```python
from build123d import *

# Parameters (mm, degrees)
BOSS_EXTRU_1_DEPTH  = 40
SKETCH1_R           = 2
CUT_EXTRUDE1_DEPTH  = 29
SKETCH2_W           = 15
SKETCH2_H           = 9
BOSS_EXTRUDE1_DEPTH = 6


with BuildPart() as part:
    # Esquisse1 → Boss.-Extru.1 (new body)
    with BuildSketch(Plane.XY):
        Polygon((0, 0), (-15, 0), (-15, -6), (0, -6), (0, -41), (-15, -41), (-15, -56), (20.126965986, -56), (20.126965986, -41), (10.126965986, -41), (10.126965986, 0), align=None)
    extrude(amount=BOSS_EXTRU_1_DEPTH)

    # Sketch1 → Cut-Extrude1 (cut)
    with BuildSketch(Plane(origin=(0, -41, 0), x_dir=(1, 0, 0), z_dir=(0, 1, 0))):
        with Locations(Location((15.126965986, -8, 0), (0, 0, 270))):
            Circle(SKETCH1_R)
        with Locations(Location((15.126965986, -32, 0), (0, 0, 270))):
            Circle(SKETCH1_R)
    extrude(amount=-CUT_EXTRUDE1_DEPTH, mode=Mode.SUBTRACT)

    # Sketch2 → Boss-Extrude1 (add)
    with BuildSketch(Plane.XY.offset(40)):
        with Locations((-7.5, -36.5)):
            Rectangle(SKETCH2_W, SKETCH2_H)
    extrude(amount=-BOSS_EXTRUDE1_DEPTH)


solid = part.part
```
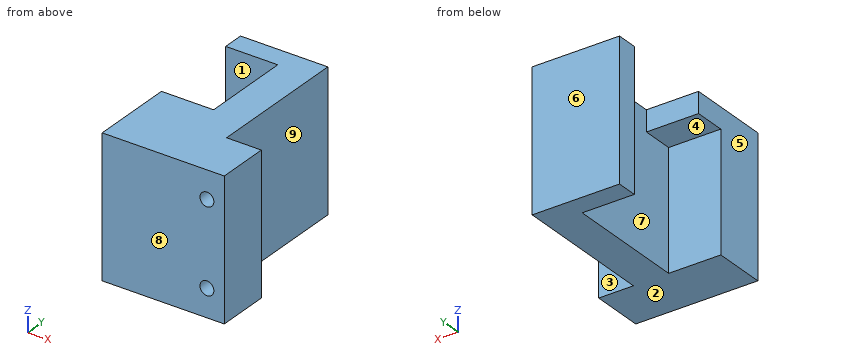
Check sheet for the modelled part. Datum: model origin and axes. Units: mm. Face numbers are marked on the shaded views. A direction names the side the tool comes from. Give positions to 0.01 mm unless a question says otherwise; leave off trailing zeros. Order: outer loops, then holes, each group sorted by start corner. A loop starts at its lowest first (then second) coordinate and runs counter-clockwise, first axis right, second up. Notation, with made-up numbers: M 8,43.5 L 34,43.5 A11 cw 34,63.5 Z; hole C 86,-8.5 d11. An arc over 180 degrees is marked long. Answer in a Markdown table with one row per item.
1) Cross-section at D-D, the plane y = -35.5. Enter the section's corners in (x, z), plus the area to 3 significant figures.
Filled sheet:
| item | result |
|---|---|
| outline | M -15,34 L 0,34 L 0,0 L 10.13,0 L 10.13,40 L -15,40 Z |
| area | 495 mm2 |
2) Cross-section at A-A, the plane x = -4.5. Enter the section's corners in (y, z), plus the area to 3 significant figures.
Filled sheet:
| item | result |
|---|---|
| outline | M -56,0 L -41,0 L -41,34 L -32,34 L -32,40 L -56,40 Z; M -6,0 L 0,0 L 0,40 L -6,40 Z |
| area | 894 mm2 |
3) Release check for a two-part mould opening along Y. For the marked faces 6, 7, 8 and 9 record: +Y half, -Y half, draft (parallel to the pull), parting line (faces both ways), or undercut.
Filled sheet:
| item | result |
|---|---|
| face 6 | +Y half |
| face 7 | undercut |
| face 8 | -Y half |
| face 9 | draft |
4) Access from +Z, -Z, +X, -X, +Y, -Y to the whole of each face (thin tool, end or side, straight path). Record for the marked faces 1, 2, 3, 4 and 5.
Filled sheet:
| item | result |
|---|---|
| face 1 | +Z, -Z, -X |
| face 2 | -Z, +X, -X, +Y, -Y |
| face 3 | +Z, -Z, +X, +Y |
| face 4 | -Z, -X |
| face 5 | +Z, -Z, -X, +Y, -Y |
5) Gauge pin test, flat ends, axial feed: P1, Ø1.5, axis at x = 12.5, z = 17.5, coming from the +Y side; P2, Ø1, axis at x = 11, y = -6.5, coming from the +Z side; P3, Ø7, axis at x = -10.5, y = -36, coming from the -Z side; P4, Ø8, axis at y = -16.5, z = 15.5, coming from the -X side. Record the tip position at first contact, or that the pin passes through.
Filled sheet:
| item | result |
|---|---|
| P1 | stops at y = -41 |
| P2 | passes through |
| P3 | stops at z = 34 |
| P4 | stops at x = 0 |
6) Thickness scan on L1, parallel to Y at x = -3, z = 5; L2, parallel to X at y = -51, z = 32; L3, parallel to Y at x = -10.5, z = 36.5. Record the ranges inside material, lowest first. Write a range as [from, to].
Filled sheet:
| item | result |
|---|---|
| L1 | y = [-56, -41], [-6, 0] |
| L2 | x = [-15, 13.13], [17.13, 20.13] |
| L3 | y = [-56, -32], [-6, 0] |
7) Cross-section at B-B, the plane z = 8. Enter the section's corners in (x, y), plus the area to 3 significant figures.
Filled sheet:
| item | result |
|---|---|
| outline | M -15,-56 L 13.13,-56 L 13.13,-41 L 10.13,-41 L 10.13,0 L -15,0 L -15,-6 L 0,-6 L 0,-41 L -15,-41 Z; M 17.13,-56 L 20.13,-56 L 20.13,-41 L 17.13,-41 Z |
| area | 972 mm2 |
8) Cross-section at C-C, the plane z = 36. Enter the section's corners in (x, y), plus the area to 3 significant figures.
Filled sheet:
| item | result |
|---|---|
| outline | M -15,-56 L 20.13,-56 L 20.13,-41 L 10.13,-41 L 10.13,0 L -15,0 L -15,-6 L 0,-6 L 0,-32 L -15,-32 Z |
| area | 1,170 mm2 |
